from build123d import *

# Parameters (mm, degrees)
SKETCH1_R           = 4
SKETCH1_R_2         = 2
BOSS_EXTRUDE1_DEPTH = 10
SKETCH2_R           = 2.5
SKETCH2_R_2         = 2
BOSS_EXTRUDE2_DEPTH = 2


with BuildPart() as part:
    # Sketch1 → Boss-Extrude1 (new body)
    with BuildSketch(Plane(origin=(0, 0, 0), x_dir=(0, 0, -1), z_dir=(1, 0, 0))):
        Circle(SKETCH1_R)
        Circle(SKETCH1_R_2, mode=Mode.SUBTRACT)
    extrude(amount=BOSS_EXTRUDE1_DEPTH)

    # Sketch2 → Boss-Extrude2 (add)
    with BuildSketch(Plane.ZY):
        Circle(SKETCH2_R)
        Circle(SKETCH2_R_2, mode=Mode.SUBTRACT)
    extrude(amount=BOSS_EXTRUDE2_DEPTH)


solid = part.part
Source: CAD feature listing. Evaluate the final solid. Frame: model axes, mm. A direction names the side the tool comes from. Give positions to 0.01 mm unless a question says otherwise; leave off trailing zeros. Write each loop counter-clockwise with the first axis right and the second up, starting at its lowest first coordinate (ties: lowest second). Pieces come first, ordered by that corner, then holes. Notation, with made-up numbers: M -25,59.5 L -13,59.5 A24 ccw -13,84.5 Z; hole C 72,30.5 d7. An arc over 180 degrees is marked long. Return JSON: item names as keys, results as strings. Group by question number.
1) Pin query (flat end, axial travel): P1, Ø1, axis at x = 5.5, z = -1.5, coming from the -Y side. Return the tip coordinate at first contact, or that it passes through.
2) Cut plane A-A, the plane y = 0. Output: boundary loops of the cut face in (x, z).
3) Set-up query: faces 1 (the face through (0, 2, -2)), 2 (the face through (4.93, -3.905, 0.867)). Return all of +Z, -Z, +X, -X, +Y, -Y with unobstructed straight access to the full face (end or side cutting, diameter ignored); none if empty.
4) Material intervals for line 1 along Y through (x, z) = (3.25, 0); line 2 along X through (y, z) = (2.5, -2); line 3 along Y through (x, z) = (-1, 1.75), sorted ascending. Write a range as [from, to].
5) Cut plane C-C, the plane x = 7.5. Output: boundary loops of the cut face in (y, z).
Recorded:
{
 "1": {"P1": "stops at y = -3.87"},
 "2": {"outline": "M -2,-2.5 L 0,-2.5 L 0,-4 L 10,-4 L 10,-2 L -2,-2 Z; M -2,2 L 10,2 L 10,4 L 0,4 L 0,2.5 L -2,2.5 Z"},
 "3": {"face 1": "-X", "face 2": "+X, -X"},
 "4": {"line 1": "y = [-4, -2], [2, 4]", "line 2": "x = [0, 10]", "line 3": "y = [-1.79, -0.97], [0.97, 1.79]"},
 "5": {"outline": "C 0,0 d8; hole C 0,0 d4"}
}
